Autodesk Inventor part; units mm, degrees
ref_plane "YZ Plane" through (0, 0, 0) normal (1, 0, 0) x (0, 1, 0)
ref_plane "XZ Plane" through (0, 0, 0) normal (0, 1, 0) x (-1, 0, 0)
ref_plane "XY Plane" through (0, 0, 0) normal (0, 0, 1) x (1, 0, 0)
sketch "Sketch1" plane through (0, 0, 0) normal (0, 1, 0) x (-1, 0, 0)
  circle A0 centre (0, 0) radius 42
  dimension "d0" = 84
extrude "Extrusion1" add sketch "Sketch1" along normal blind 50
sketch "Sketch3" plane through (0, 0, 0) normal (1, 0, 0) x (0, 1, 0)
  line L0 (50, -42) -> (50, 42)
  circle A0 centre (50, -16) radius 9
  line L1 (-11.8, 0) -> (70.8, 0)
  line L2 (71.2036, 0) -> (0, 0)
  point P0 (50, -7)
  point P1 (50, -25)
  dimension "d4" = 18
  dimension "d5" = 32
revolve "Revolution1" cut sketch "Sketch3" angle 360 about axis through (0, -10, 0) along (0, 1, 0) picked at (45.6277, -15.2948) contours A0 L0
sketch "Sketch4" plane through (0, 0, 0) normal (1, 0, 0) x (0, 1, 0)
  line L0 (0, -42) -> (0, 42)
  line L1 (0, -20) -> (25, -20)
  line L2 (25, -20) -> (25, -95.9961)
  line L3 (25, -95.9961) -> (0, -95.9961)
  line L4 (0, -95.9961) -> (0, -20)
  line L5 (-10, 0) -> (60, 0)
  line L6 (0, 20) -> (25, 20)
  line L7 (25, 20) -> (25, 95.9961)
  line L8 (25, 95.9961) -> (0, 95.9961)
  line L9 (0, 95.9961) -> (0, 20)
  point P0 (0, 0)
  dimension "d7" = 25
  dimension "d8" = 20
extrude "Extrusion2" cut sketch "Sketch4" along normal mid plane 100
shell "Shell1" thickness 5 removed faces 1 at (11.381, 0, 4.5482)
properties material "Aluminum 6061"
Source: CAD feature listing. Evaluate the final solid. Frame: model axes, mm. A direction names the side the tool comes from. Give positions to 0.01 mm unless a question says otherwise; leave off trailing zeros. Write each loop counter-clockwise with the first axis right and the second up, starting at its lowest first coordinate (ties: lowest second). Pieces come first, ordered by that corner, then holes. Notation, with made-up numbers: (34.25, 22) - (48.25, 22) arc R22 ccw to (48.25, 37) - close; hole circle Ø8 at (68, 59.25). An arc over 180 degrees is marked (long way). One line per item, written item: value. Start each with the question number.
Q1. Material intervals for probe 1 along Z at (x, y) = (0, 16.5); probe 2 along X at (y, z) = (34, 0); probe 3 along Z at (x, y) = (0, 27), sorted ascending. Write a range as from..to.
Q2. Section query B-B, the plane z = 0. Return the cut outline in (x, y).
Q3. First-contact query: pin 1 Ø1.5 at (x, y) = (-32, 38) entering from -Z; pin 2 Ø1 at (x, y) = (17, 34) entering from +Z; pin 3 Ø4.5 at (x, z) = (1, -1.5) entering from -Y; pin 4 Ø8 at (y, z) = (9.5, -26.5) entering from -X. Flat tips, straight axial feed; report the tip coordinate or a pass-through.
Q4. Set-up query: faces 1 (the face through (-1, 12, 20)), 2 (the face through (-1, 25, -28)), 3 (the face through (0, 50, 0)), 4 (the face through (0, 30, -23)), 5 (the face through (0, 15, 15)). Return all of +Z, -Z, +X, -X, +Y, -Y with unobstructed straight access to the full face (end or side cutting, diameter ignored); none if empty.
Q5. Section query A-A, the plane y = 4. Return the cut outline in (x, z), then the cut area to 3 significant figures.
Q6. Section query C-C, the plane x = 0. Return the cut outline in (y, z).
Q7. Draft query along X for faces 6 (the face through (-1, 12, -20)), 7 (the face through (-16.3, 45, -24.5)), 8 (the face through (-40.06, 30.21, -12.62)), 9 (the face through (0, 15, -15)). Return one class per face: +X half, -X half, draft (parallel to the pull), parting line (faces both ways), or undercut.
Q8. Section query D-D, the plane z = -34. Return the cut outline in (x, y), then the cut area to 3 significant figures.
Answer:
1. probe 1: z = -20..-15, 15..20
1. probe 2: x = -42..-37, 37..42
1. probe 3: z = -42..-15, 15..42
2. outline: (-42, 0) - (-37, 0) - (-37, 45) - (-29.08, 45) arc R14 ccw to (-2.92, 45) - (2.92, 45) arc R14 ccw to (29.08, 45) - (37, 45) - (37, 0) - (42, 0) - (42, 50) - (25, 50) arc R9 cw to (7, 50) - (-7, 50) arc R9 cw to (-25, 50) - (-42, 50) - close
3. pin 1: stops at z = -28.06
3. pin 2: stops at z = 38.62
3. pin 3: stops at y = 42.7
3. pin 4: passes through
4. face 1: +Z, +X, -X, -Y
4. face 2: -Z, +X, -X, -Y
4. face 3: +Z, -Z, +X, -X, +Y
4. face 4: none
4. face 5: -Y
5. outline: (-36.93, -20) - (36.93, -20) arc R42 ccw to (36.93, 20) - (-36.93, 20) arc R42 ccw to start; hole (-33.82, -15) - (33.82, -15) arc R37 ccw to (33.82, 15) - (-33.82, 15) arc R37 ccw to start
5. area: 1,070 mm2
6. outline: (0, -20) - (25, -20) - (25, -42) - (50, -42) - (50, -25) arc R9 cw to (50, -7) - (50, 7) arc R9 cw to (50, 25) - (50, 42) - (25, 42) - (25, 20) - (0, 20) - (0, 15) - (30, 15) - (30, 37) - (45, 37) - (45, 29.08) arc R14 ccw to (45, 2.92) - (45, -2.92) arc R14 ccw to (45, -29.08) - (45, -37) - (30, -37) - (30, -15) - (0, -15) - close
7. face 6: draft
7. face 7: undercut
7. face 8: parting line
7. face 9: undercut
8. outline: (-24.66, 25) - (24.66, 25) - (24.66, 50) - (-24.66, 50) - close; hole (-14.59, 30) - (14.59, 30) - (14.59, 45) - (-14.59, 45) - close
8. area: 795 mm2
